```python
from build123d import *

# Parameters (mm, degrees)
EXTRUDE_1_DEPTH        = 31.5
EXTRUDE_1_DEPTH_BACK   = 31.5
CHAMFER_1_SIZE         = 12
CHAMFER_1_SIZE2        = 17.137776081
EXTRUDE_1_2_DEPTH      = 2
EXTRUDE_2_DEPTH        = 2
FILLET_1_R             = 0.7
FILLET_1_OF_MIRROR_1_R = 0.7


with BuildPart() as part:
    # 草图1 → Extrude 1 (new, two sides: drawn at the far end of the back side and taken through both)
    with BuildSketch(Plane(origin=(0, 0, 0), x_dir=(1, 0, 0), z_dir=(0, 1, 0)).offset(-EXTRUDE_1_DEPTH_BACK)):
        Polygon((0, -8), (0, 8), (-17.240931671, 20.67715564), (-51.420742101, 20.67715564), (-51.420742101, 23.17715564), (-16.420742101, 23.17715564), (2.5, 9.264845271), (2.5, -8.950498306), (-6.131476703, -18.660909597), (-8, -17), align=None)
    extrude(amount=EXTRUDE_1_DEPTH + EXTRUDE_1_DEPTH_BACK)

    # 倒角1
    chamfer_1_edges = [part.edges().sort_by_distance(p)[0] for p in [
        (-51.420742101, -31.5, -21.92715564),
        (-51.420742101, 31.5, -21.92715564),
    ]]
    chamfer_1_side = [part.faces().sort_by_distance(p)[0] for p in [
        (-51.420742101, 0, -21.92715564),
    ]]
    chamfer(chamfer_1_edges, length=CHAMFER_1_SIZE, length2=CHAMFER_1_SIZE2, reference=chamfer_1_side[0])

    # 草图4 → Extrude 1 2 (add)
    with BuildSketch(Plane(origin=(0, 10.5, 0), x_dir=(1, 0, 0), z_dir=(0, 1, 0))):
        Polygon((-6.131476703, -18.660909597), (2.5, -8.950498306), (2.5, 9.264845271), (-16.420742101, 23.17715564), (-34.282966021, 23.17715564), (-51.420742101, 23.17715564), (-51.420742101, 13.17715564), (-34.282966021, 13.17715564), (-19.701500378, 13.17715564), (-7.5, 4.205464186), (-7.5, -5.148505082), (-13.60556989, -12.017271209), align=None)
        Polygon((-5.010362725, -19.657455355), (4, -9.520797289), (4, 10.023752434), (-15.92862836, 24.67715564), (-34.282966021, 24.67715564), (-51.420742101, 24.67715564), (-51.420742101, 14.67715564), (-34.282966021, 14.67715564), (-19.209386637, 14.67715564), (-6, 4.964371348), (-6, -5.718804066), (-12.484455912, -13.013816967), align=None)
    extrude_1_2 = extrude(amount=-EXTRUDE_1_2_DEPTH)

    # 草图5 → 拉伸-薄壁2 (add)
    with BuildSketch(Plane(origin=(0, 14.5, 0), x_dir=(1, 0, 0), z_dir=(0, 1, 0))):
        Polygon((-6.131476703, -18.660909597), (2.5, -8.950498306), (2.5, 9.264845271), (-16.420742101, 23.17715564), (-34.282966021, 23.17715564), (-51.420742101, 23.17715564), (-51.420742101, 13.17715564), (-34.282966021, 13.17715564), (-19.701500378, 13.17715564), (-7.5, 4.205464186), (-7.5, -5.148505082), (-13.60556989, -12.017271209), align=None)
        Polygon((-5.010362725, -19.657455355), (4, -9.520797289), (4, 10.023752434), (-15.92862836, 24.67715564), (-34.282966021, 24.67715564), (-51.420742101, 24.67715564), (-51.420742101, 14.67715564), (-34.282966021, 14.67715564), (-19.209386637, 14.67715564), (-6, 4.964371348), (-6, -5.718804066), (-12.484455912, -13.013816967), align=None)
    extrude_2 = extrude(amount=-EXTRUDE_2_DEPTH)

    # 圆角1
    fillet_1_edges = [part.edges().sort_by_distance(p)[0] for p in [
        (-33.674685231, 12.5, -24.67715564),
        (-5.96431418, 12.5, -17.350454037),
        (4, 12.5, -0.251477572),
        (-0.505181363, 12.5, 14.589126322),
        (-33.674685231, 14.5, -24.67715564),
        (-5.96431418, 14.5, -17.350454037),
        (4, 14.5, -0.251477572),
        (-0.505181363, 14.5, 14.589126322),
        (-33.674685231, 8.5, -24.67715564),
        (-5.96431418, 8.5, -17.350454037),
        (4, 8.5, -0.251477572),
        (-0.505181363, 8.5, 14.589126322),
        (-33.674685231, 10.5, -24.67715564),
        (-5.96431418, 10.5, -17.350454037),
        (4, 10.5, -0.251477572),
        (-0.505181363, 10.5, 14.589126322),
    ]]
    fillet(fillet_1_edges, radius=FILLET_1_R)

    # 镜向1: Extrude 1 2, 拉伸-薄壁2 across plane
    add(extrude_1_2.mirror(Plane.ZX))
    add(extrude_2.mirror(Plane.ZX))

    # 圆角1 of 镜向1
    fillet_1_of_mirror_1_edges = [part.edges().sort_by_distance(p)[0] for p in [
        (-33.674685231, -12.5, -24.67715564),
        (-5.96431418, -12.5, -17.350454037),
        (4, -12.5, -0.251477572),
        (-0.505181363, -12.5, 14.589126322),
        (-33.674685231, -14.5, -24.67715564),
        (-5.96431418, -14.5, -17.350454037),
        (4, -14.5, -0.251477572),
        (-0.505181363, -14.5, 14.589126322),
        (-33.674685231, -8.5, -24.67715564),
        (-5.96431418, -8.5, -17.350454037),
        (4, -8.5, -0.251477572),
        (-0.505181363, -8.5, 14.589126322),
        (-33.674685231, -10.5, -24.67715564),
        (-5.96431418, -10.5, -17.350454037),
        (4, -10.5, -0.251477572),
        (-0.505181363, -10.5, 14.589126322),
    ]]
    fillet(fillet_1_of_mirror_1_edges, radius=FILLET_1_OF_MIRROR_1_R)


solid = part.part
```
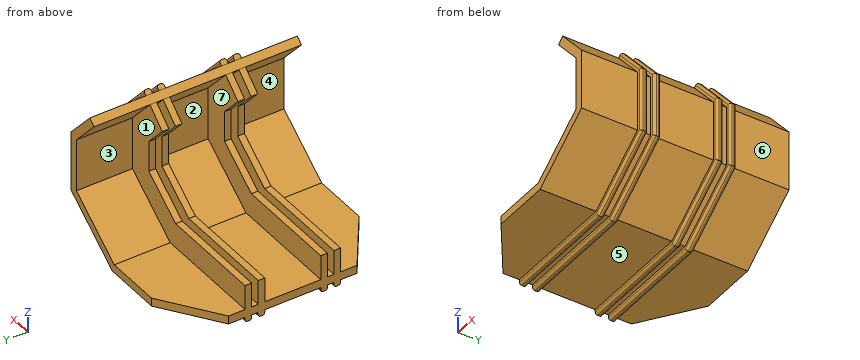
For this review, take the finished solid that the model builds, in its own axes (mm). Face numbers are marked on the shaded views. A direction names the side the tool comes from. Coordinates: 2 decimals unless noted, no trailing zeros. Loops run counter-clockwise (first coordinate to the right, second up) from the corner with the lowest first, then second, coordinate; pieces in that order, holes last. Notation, with made-up numbers: (0.5, -25.75) - (40.5, -25.75) arc R21 ccw to (40.5, -15.75) - close; hole circle Ø10 at (38.5, 12.25). An arc over 180 degrees is marked (long way). Use one line per item in the form item = value. Start each with the question number.
1) Take a section at C-C (y = -22.5). State the section outline as (x, z) points.
2) Draft analysis for pull direction Y (two halves, no side actions). For the marked faces 1, 2 and 3, state which applies: released by +Y, released by -Y, zero draft, split by the parting line, or undercut.
3) To check wall thickness, follow probe 1 along Y at (x, z) = (-33.5, -20.5); probe 2 along Z at (x, y) = (-28.5, -20); probe 3 along X at (y, z) = (-1, -7.5). State the ranges of each line that lie inside material, in increasing order. Write a range as from..to.
4) For pin 1 (2 mm diameter, centred on y = 12, z = 4.5, fed in from +X); pin 2 (13 mm diameter, centred on y = -23.5, z = 2, fed in from -X); pin 3 (1.6 mm diameter, centred on x = -39.5, y = 12, fed in from -Z), all flat-tipped, find the tip position at first contact; note any pin that passes through.
5) For the marked faces 4, 5, 6 and 7, list the 3-axis set-ups (+Z, -Z, +X, -X, +Y, -Y) from which the entire face can be reached by the end or side of a thin tool; tool diameter is ignored.
6) Take a section at A-A (y = -4.5). State the section outline as (x, z) points, plus the area to 3 significant figures.
7) Take a section at B-B (x = -12). State how many separate pieces and enclosed holes the cut face has, plus the area to 3 significant figures.
From the geometry:
q1.outline = (-47.14, -23.18) - (-16.42, -23.18) - (2.5, -9.26) - (2.5, 8.95) - (-6.13, 18.66) - (-8, 17) - (0, 8) - (0, -8) - (-17.24, -20.68) - (-47.14, -20.68) - close
q2.face_1 = released by +Y
q2.face_2 = undercut
q2.face_3 = zero draft
q3.probe_1 = -14.5..-12.5, -10.5..-8.5, 8.5..10.5, 12.5..14.5
q3.probe_2 = -23.18..-20.68
q3.probe_3 = 0..2.5
q4.pin_1 = 3.97
q4.pin_2 = -0.44
q4.pin_3 = -24.55
q5.face_4 = -X, -Y
q5.face_5 = -Z, +X, -X
q5.face_6 = +Z, -Z, +X, +Y
q5.face_7 = -X
q6.outline = (-51.42, -23.18) - (-16.42, -23.18) - (2.5, -9.26) - (2.5, 8.95) - (-6.13, 18.66) - (-8, 17) - (0, 8) - (0, -8) - (-17.24, -20.68) - (-51.42, -20.68) - close
q6.area = 217 mm2
q7.separate_pieces = 5
q7.enclosed_holes = 0
q7.area = 310 mm2
